from build123d import *

# Parameters (mm, degrees)
F1_DEPTH = 50
F3_DEPTH = 30
F4_R     = 5


with BuildPart() as f1:
    # F0 (on Top) → F1 (new body)
    with BuildSketch(Plane.XY):
        Polygon((0, 40), (-70, 40), (-70, -40), (0, -40), (0, 0), align=None)
        Polygon((70, 40), (0, 40), (0, 0), (0, -40), (70, -40), align=None)
    extrude(amount=F1_DEPTH)

    # F2 (on face) → F3 (join)
    with BuildSketch(Plane.XY.offset(50)):
        with BuildLine():
            Line((-70, 40), (-70, 15))
            Line((-70, 15), (-50, 15))
            ThreePointArc((-50, 15), (-46.464466, 16.464466), (-45, 20))
            Line((-45, 20), (-45, 40))
            Line((-45, 40), (-70, 40))
        make_face()
    extrude(amount=F3_DEPTH)

    # F4
    f4_edges = [f1.edges().sort_by_distance(p)[0] for p in [
        (-70, 40, 40),
    ]]
    fillet(f4_edges, radius=F4_R)


solid = f1.part
Geometry check sheet. Reference: the model listing, model coordinates, mm. A direction names the side the tool comes from. Round coordinates to 2 decimals unless told otherwise and drop trailing zeros. Order: outer loops, then holes, each group sorted by start corner. A loop starts at its lowest first (then second) coordinate and runs counter-clockwise, first axis right, second up. Notation, with made-up numbers: M -30,0 L -17,0 A34 cw -17,38 Z; hole C 3,9.25 d5. An arc over 180 degrees is marked long. Answer in a Markdown table with one row per item.
(1) Tool access check on faces 1 (the face through (-60, 15, 65)), 2 (the face through (-45, 30, 65)), 3 (the face through (-1, 1, 50)). Record the directions out of +Z, -Z, +X, -X, +Y, -Y that give a thin tool (end or side, any length) a straight path to the whole face; none if there is none.
Responses:
| item | result |
|---|---|
| face 1 | +Z, +X, -X, -Y |
| face 2 | +Z, +X, +Y, -Y |
| face 3 | +Z, +X, -Y |
(2) Go/stop test with flat-tipped pins: P1, Ø1, axis at x = 8.5, y = -29.5, coming from the +Z side; P2, Ø1, axis at x = -42, z = 52, coming from the -Y side; P3, Ø6, axis at y = 33, z = 60, coming from the +X side; P4, Ø16, axis at x = -57, z = 65.5, coming from the -Y side. Record where each tip stops, or that it passes through.
Responses:
| item | result |
|---|---|
| P1 | stops at z = 50 |
| P2 | passes through |
| P3 | stops at x = -45 |
| P4 | stops at y = 15 |
(3) Scan lines: probe 1 along Z at (x, y) = (11, 33.5); probe 2 along X at (y, z) = (25, 72.5); probe 3 along Y at (x, z) = (-57, 59.5). Record each from-to range of solid material in increasing order. Write a range as from..to.
Responses:
| item | result |
|---|---|
| probe 1 | z = 0..50 |
| probe 2 | x = -70..-45 |
| probe 3 | y = 15..40 |
(4) Sectioned sample at A-A, the plane y = 30. Record the cut outline in (x, z), and give its area (3 significant figures).
Responses:
| item | result |
|---|---|
| outline | M -70,0 L 70,0 L 70,50 L -45,50 L -45,80 L -70,80 Z |
| area | 7,750 mm² |
(5) Sectioned sample at C-C, the plane x = 39. Record the cut outline in (y, z), and give its area (3 significant figures).
Responses:
| item | result |
|---|---|
| outline | M -40,0 L 40,0 L 40,50 L -40,50 Z |
| area | 4,000 mm² |
(6) Sectioned sample at D-D, the plane y = -18.5. Record the cut outline in (x, z), and give its area (3 significant figures).
Responses:
| item | result |
|---|---|
| outline | M -70,0 L 70,0 L 70,50 L -70,50 Z |
| area | 7,000 mm² |
(7) Sectioned sample at B-B, the plane z = 58. Record the cut outline in (x, y), and give its area (3 significant figures).
Responses:
| item | result |
|---|---|
| outline | M -70,15 L -50,15 A5 ccw -45,20 L -45,40 L -65,40 A5 ccw -70,35 Z |
| area | 614 mm² |
